from build123d import *

# Parameters (mm, degrees)
SKETCH_R        = 9
PAD_DEPTH       = 65
SKETCH001_W     = 6
SKETCH001_H     = 6
PAD001_DEPTH    = 1
SKETCH002_R     = 1.15
POCKET_DEPTH    = 5
SKETCH003_W     = 6
SKETCH003_H     = 6
PAD002_DEPTH    = 1
SKETCH004_R     = 1.15
POCKET001_DEPTH = 5


with BuildPart() as part:
    # Sketch → Pad (new body)
    with BuildSketch(Plane.XY):
        Circle(SKETCH_R)
    extrude(amount=PAD_DEPTH)

    # Sketch001 (on Face3 of Pad) → Pad001 (join)
    with BuildSketch(Plane.XY.offset(65)):
        Rectangle(SKETCH001_W, SKETCH001_H)
    extrude(amount=PAD001_DEPTH)

    # Sketch002 (on Face8 of Pad001) → Pocket (cut)
    with BuildSketch(Plane.XY.offset(66)):
        Circle(SKETCH002_R)
    extrude(amount=-POCKET_DEPTH, mode=Mode.SUBTRACT)

    # Sketch003 (on Face2 of Pocket) → Pad002 (join)
    with BuildSketch(Plane(origin=(0, 0, 0), x_dir=(1, 0, 0), z_dir=(0, 0, -1))):
        Rectangle(SKETCH003_W, SKETCH003_H)
    extrude(amount=PAD002_DEPTH)

    # Sketch004 (on Face12 of Pad002) → Pocket001 (cut)
    with BuildSketch(Plane(origin=(0, 0, -1), x_dir=(1, 0, 0), z_dir=(0, 0, -1))):
        Circle(SKETCH004_R)
    extrude(amount=-POCKET001_DEPTH, mode=Mode.SUBTRACT)


solid = part.part
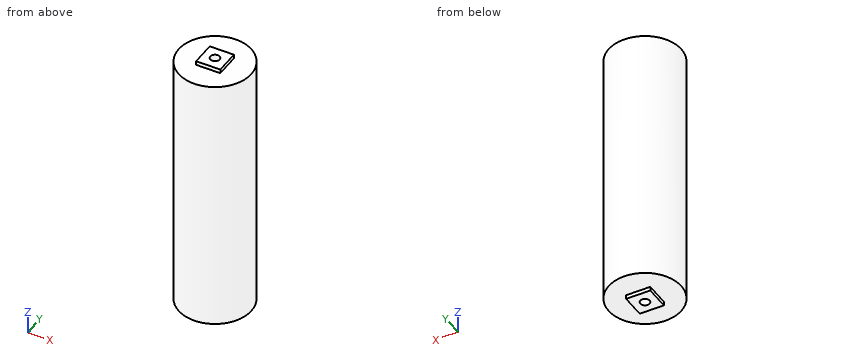
Input: part model. Units: mm. Frame: model coordinates. Coordinates: 2 decimals unless noted, no trailing zeros. Loops run counter-clockwise (first coordinate to the right, second up) from the corner with the lowest first, then second, coordinate; pieces in that order, holes last.
(1) Section D-D on y = 5.5. Return the cut outline in (x, z), then the cut area to 3 significant figures.
(2) Material intervals for probe 1 along Y at (x, z) = (0, 2.2); probe 2 along Z at (x, y) = (-0.25, 6); probe 3 along Z at (x, y) = (0.5, 0), sorted ascending.
(3) Section C-C on z = 9.5. Return the cut outline in (x, y), then the cut area to 3 significant figures.
(4) Section A-A on y = 0. Return the cut outline in (x, z).
(5) First-contact query: pin 1 Ø8 at (x, z) = (5, 16) entering from -Y; pin 2 Ø3 at (x, z) = (-5.5, 33.5) entering from +Y; pin 3 Ø1.2 at (x, y) = (0, 0) entering from -Z. Flat tips, straight axial feed; report the tip coordinate or a pass-through.
Data:
1. outline: (-7.12, 0) - (7.12, 0) - (7.12, 65) - (-7.12, 65) - close
1. area: 926 mm2
2. probe 1: y = -9 to -1.15, 1.15 to 9
2. probe 2: z = 0 to 65
2. probe 3: z = 4 to 61
3. outline: circle Ø18 at (0, 0)
3. area: 254 mm2
4. outline: (-9, 0) - (-3, 0) - (-3, -1) - (-1.15, -1) - (-1.15, 4) - (1.15, 4) - (1.15, -1) - (3, -1) - (3, 0) - (9, 0) - (9, 65) - (3, 65) - (3, 66) - (1.15, 66) - (1.15, 61) - (-1.15, 61) - (-1.15, 66) - (-3, 66) - (-3, 65) - (-9, 65) - close
5. pin 1: stops at y = -8.94
5. pin 2: stops at y = 8.06
5. pin 3: stops at z = 4
